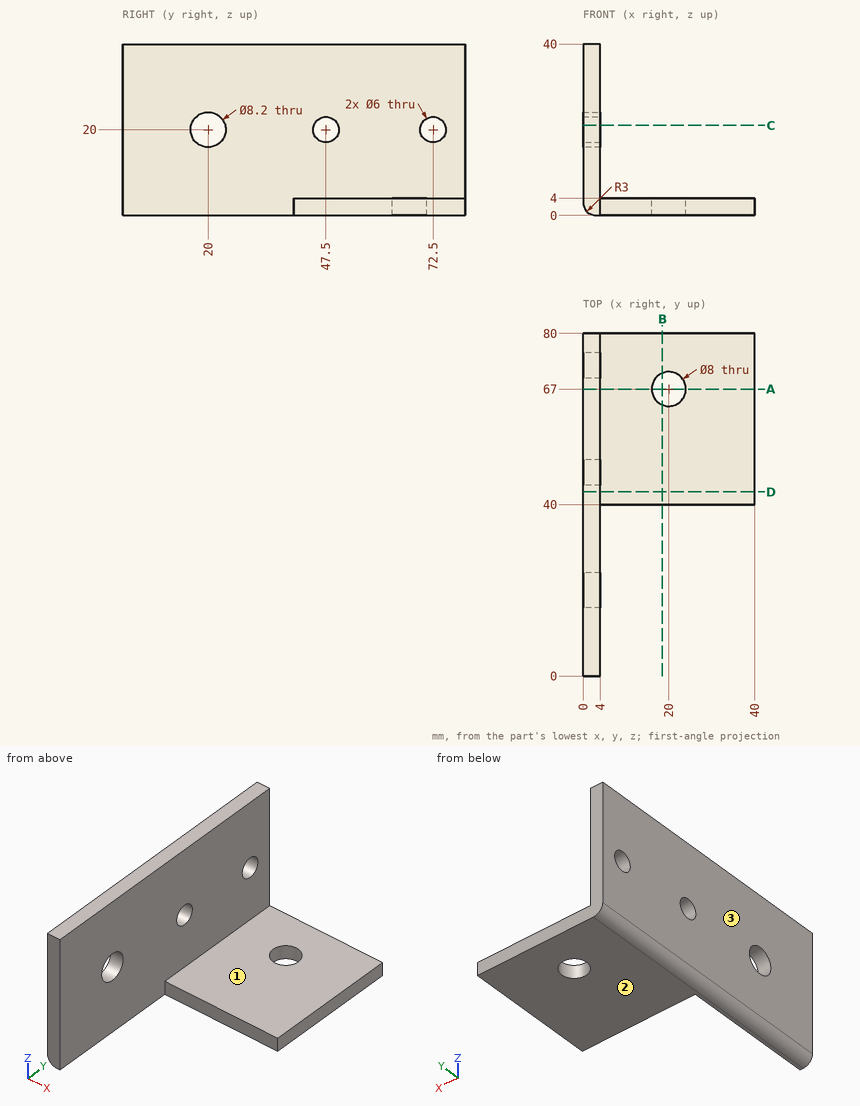
Geometry check sheet. Reference: drawing and pictorial views, mm from the part's lowest x, y, z. Give positions to 0.01 mm unless a question says otherwise; leave off trailing zeros. Order: outer loops, then holes, each group sorted by start corner. A loop starts at its lowest first (then second) coordinate and runs counter-clockwise, first axis right, second up. Notation, with made-up numbers: (27, 18.5) - (77, 18.5) arc R10 ccw to (77, 23.5) - close; hole circle Ø6 at (64, -3.75). An arc over 180 degrees is marked (long way). Use one line per item in the form item = value.
1) Sectioned sample at B-B (x = 18.5). Record the boundary of the cut face in (y, z), and give its area (3 significant figures).
Working result:
outline = (40, 0) - (63.29, 0) - (63.29, 4) - (40, 4) - close; (70.71, 0) - (80, 0) - (80, 4) - (70.71, 4) - close
area = 130 mm^2
2) Material ranges on probe 1 along Y at (x, z) = (1.4, 20); probe 2 along Y at (x, z) = (20, 3); probe 3 along X at (y, z) = (62, 23.5), recorded low to high. Write a range as from..to.
Working result:
probe_1 = 0..15.9, 24.1..44.5, 50.5..69.5, 75.5..80
probe_2 = 40..63, 71..80
probe_3 = 0..4
3) Sectioned sample at A-A (y = 67). Record the boundary of the cut face in (x, z), and give its area (3 significant figures).
Working result:
outline = (0, 3) arc R3 ccw to (3, 0) - (16, 0) - (16, 4) - (4, 4) - (4, 40) - (0, 40) - close; (24, 0) - (40, 0) - (40, 4) - (24, 4) - close
area = 270 mm^2
4) Sectioned sample at D-D (y = 43). Record the boundary of the cut face in (x, z), and give its area (3 significant figures).
Working result:
outline = (0, 3) arc R3 ccw to (3, 0) - (40, 0) - (40, 4) - (4, 4) - (4, 40) - (0, 40) - close
area = 302 mm^2
5) Draft check along Z on the marked faces 1, 2 and 3. Enter one of: released by +Z, released by -Z, zero draft, split by the parting line, or undercut.
Working result:
face_1 = released by +Z
face_2 = released by -Z
face_3 = zero draft
6) Depth check by flat-ended pin: pin 1 Ø1.5 at (x, y) = (28, 67) entering from +Z; pin 2 Ø5 at (y, z) = (47.5, 20) entering from +X; pin 3 Ø1.2 at (x, z) = (23.5, 2.5) entering from -Y; pin 4 Ø12 at (y, z) = (35.5, 30) entering from +X. Enter the tip coordinate at first touch or a pass-through.
Working result:
pin_1 = 4
pin_2 = through
pin_3 = 40
pin_4 = 4
7) Sectioned sample at C-C (z = 21). Record the boundary of the cut face in (x, y).
Working result:
outline = (0, 0) - (4, 0) - (4, 16.02) - (0, 16.02) - close; (0, 23.98) - (4, 23.98) - (4, 44.67) - (0, 44.67) - close; (0, 50.33) - (4, 50.33) - (4, 69.67) - (0, 69.67) - close; (0, 75.33) - (4, 75.33) - (4, 80) - (0, 80) - close
